The listing builds one solid part. Answer for the finished solid, in the listing's coordinates (mm). A direction names the side the tool comes from. Round coordinates to 2 decimals unless told otherwise and drop trailing zeros. Write each loop counter-clockwise with the first axis right and the second up, starting at its lowest first coordinate (ties: lowest second). Pieces come first, ordered by that corner, then holes. Notation, with made-up numbers: (26.25, 85.5) - (85.25, 85.5) arc R26 cw to (85.25, 119.5) - close; hole circle Ø11 at (-30, 45). An arc over 180 degrees is marked (long way). Answer as CSV lines item,"result". Start each with the question number.
Item 1: Straight lines are drawn through the part: line 1 along Z through (x, y) = (26.5, 0); line 2 along Z through (x, y) = (31, 0); line 3 along Z through (x, y) = (5.5, 0). For each, find the intervals that lie inside material, in ascending order. Write a range as [from, to].
Item 2: A cutting plane is placed at C-C on x = 34.5. Determine the outline of the cut face in (y, z), and give its area (3 significant figures).
Item 3: A cutting plane is placed at A-A on x = 2.5. Determine the outline of the cut face in (y, z).
Item 4: For a pull along Y with two mould halves and no side action, classify faces 4 (the conical face through (20.78, -9.65, -43.45)), 5 (the flat face through (0, 4, 21)), 6 (the cylindrical face through (26.031, -3.243, -33.979)), 7 (the conical face through (13.062, 0.128, -35.576)) as pulls with the +Y half, pulls with the -Y half, needs draft (parallel to the pull), parting line crosses it, or undercut.
Item 5: Which of the six approach directions +Z, -Z, +X, -X, +Y, -Y give full straight-line access (tool end or side, diameter ignored) to faces 1 (the cylindrical face through (26.03, 31.63, 0.44)), 2 (the flat face through (37, -18.9, 20.2)), 3 (the flat face through (5, -21, -19))?
Item 6: Flat-ended cylindrical pins translate along their axes: pin 1 (1 mm diameter, centred on x = 16.5, z = 28, fed in from +Y); pin 2 (3 mm diameter, centred on x = 13.5, z = 25.5, fed in from -Y); pin 3 (10 mm diameter, centred on y = -30.5, z = -23.5, fed in from -X); pin 4 (10 mm diameter, centred on y = 22.5, z = 5, fed in from +X). Find the tip coordinate at first contact, or state that the pin passes through.
Item 7: A cutting plane is placed at B-B on x = 28. Determine the outline of the cut face in (y, z), and give its area (3 significant figures).
```python
from build123d import *

# Parameters (mm, degrees)
DAIRESEL_KAPLAMA2_COUNT = 4


with BuildPart() as part:
    # Çizim1 → Döndür1 (revolve)
    with BuildSketch(Plane.XY):
        Polygon((0, 21), (11, 21), (11, 27.5), (37, 27.5), (37, 44), (5, 45), (5, 28), (0, 28), align=None)
    revolve(axis=Axis((0, 0, 0), (1, 0, 0)))

    # Çizim4 → M8 Dişli Delik1 (revolve, cut)
    with BuildSketch(Plane(origin=(37, 35, 0), x_dir=(0, 0, -1), z_dir=(0, 1, 0))):
        Polygon((0, 0), (0, 24.292926105), (3.4, 22.25), (3.4, 0), align=None)
    m8_di_li_delik1 = revolve(axis=Axis((43.35, 35, 0), (-1, 0, 0)), mode=Mode.SUBTRACT)

    # Dairesel Kaplama2: M8 Dişli Delik1 ×4 about axis
    dairesel_kaplama2_axis = Axis((0, 0, 0), (1, 0, 0))
    for i in range(1, DAIRESEL_KAPLAMA2_COUNT):
        add(m8_di_li_delik1.rotate(dairesel_kaplama2_axis, i * 360 / DAIRESEL_KAPLAMA2_COUNT), mode=Mode.SUBTRACT)


solid = part.part
```
Geometry says:
1,line 1,"z = [-44.33, -38.4], [-31.6, -27.5], [27.5, 31.6], [38.4, 44.33]"
1,line 2,"z = [-44.19, -38.4], [-31.6, -27.5], [27.5, 31.6], [38.4, 44.19]"
1,line 3,"z = [-44.98, -21], [21, 44.98]"
2,outline,"circle Ø88.16 at (0, 0); hole circle Ø6.8 at (-35, 0); hole circle Ø55 at (0, 0); hole circle Ø6.8 at (0, -35); hole circle Ø6.8 at (0, 35); hole circle Ø6.8 at (35, 0)"
2,area,"3,580 mm^2"
3,outline,"circle Ø56 at (0, 0); hole circle Ø42 at (0, 0)"
4,face 4,"parting line crosses it"
4,face 5,"needs draft"
4,face 6,"undercut"
4,face 7,"undercut"
5,face 1,"+X"
5,face 2,"+Z, -Z, +X, +Y, -Y"
5,face 3,"-X"
6,pin 1,"stops at y = 35.16"
6,pin 2,"stops at y = -37.75"
6,pin 3,"stops at x = 5"
6,pin 4,"stops at x = 37"
7,outline,"circle Ø88.56 at (0, 0); hole circle Ø6.8 at (-35, 0); hole circle Ø55 at (0, 0); hole circle Ø6.8 at (0, -35); hole circle Ø6.8 at (0, 35); hole circle Ø6.8 at (35, 0)"
7,area,"3,640 mm^2"
